Can you work these out from the model? Positions are in its coordinate system, mm. Face numbers are marked on the shaded views. A direction names the side the tool comes from. Coordinates: 2 decimals unless noted, no trailing zeros. Order: outer loops, then holes, each group sorted by start corner. A loop starts at its lowest first (then second) coordinate and runs counter-clockwise, first axis right, second up. Notation, with made-up numbers: (-18.5, -26) -> (5.5, -26) arc R14 ccw to (5.5, -8) -> close; hole circle Ø1 at (-25.5, 56.5). An arc over 180 degrees is marked (long way). Write item = value, one per line.
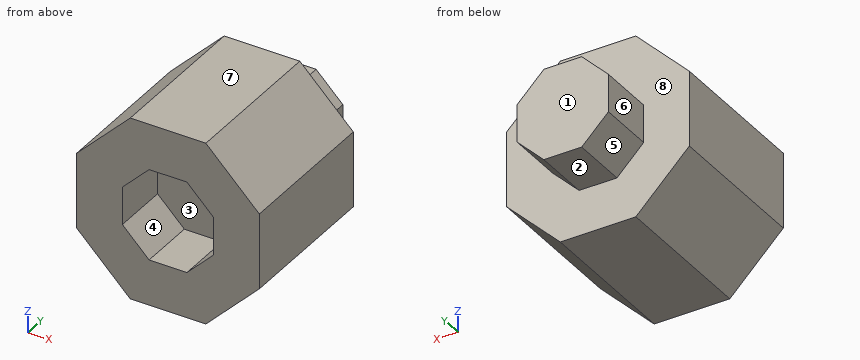
```python
from build123d import *

# Parameters (mm, degrees)
F1_DEPTH = 40
F3_DEPTH = 15
F5_DEPTH = 15


with BuildPart() as f1:
    # F0 (on Front) → F1 (new body)
    with BuildSketch(Plane.XZ):
        Polygon((24, -9.941125497), (24, 9.941125497), (9.941125497, 24), (-9.941125497, 24), (-24, 9.941125497), (-24, -9.941125497), (-9.941125497, -24), (9.941125497, -24), align=None)
    extrude(amount=F1_DEPTH)

    # F2 (on Front) → F3 (join)
    with BuildSketch(Plane.XZ):
        Polygon((4.9705627485, -12), (12, -4.9705627485), (12, 4.9705627485), (4.9705627485, 12), (-4.9705627485, 12), (-12, 4.9705627485), (-12, -4.9705627485), (-4.9705627485, -12), align=None)
    extrude(amount=-F3_DEPTH)

    # F4 (on face) → F5 (cut)
    with BuildSketch(Plane.XZ.offset(40)):
        Polygon((-4.9705627485, -12), (4.9705627485, -12), (12, -4.9705627485), (12, 4.9705627485), (4.9705627485, 12), (-4.9705627485, 12), (-12, 4.9705627485), (-12, -4.9705627485), align=None)
    extrude(amount=-F5_DEPTH, mode=Mode.SUBTRACT)


solid = f1.part
```
Item 1: For the marked faces 4, 5, 6, 7 and 8, which set-ups out of +Z, -Z, +X, -X, +Y, -Y let a thin tool reach every point of the face, with its end or its side?
A:
face_4 = -Y
face_5 = -Z, -X, +Y
face_6 = +Z, -Z, -X, +Y
face_7 = +Z, +X, -X, +Y, -Y
face_8 = +Y
Item 2: I want a section at B-B, the plane x = 1. Please give me the cut outline in (y, z), plus the area to 3 significant figures.
A:
outline = (-40, -24) -> (0, -24) -> (0, -12) -> (15, -12) -> (15, 12) -> (0, 12) -> (0, 24) -> (-40, 24) -> (-40, 12) -> (-25, 12) -> (-25, -12) -> (-40, -12) -> close
area = 1,920 mm2
Item 3: If we mould it in two halves opening along Z, with no side actions, what happens to the marked faces 1, 2 and 3? For each: pulls with the +Z half, pulls with the -Z half, needs draft (parallel to the pull), parting line crosses it, or undercut.
A:
face_1 = needs draft
face_2 = pulls with the -Z half
face_3 = undercut
Item 4: I'm going to push flat-ended pins straight in: P1, Ø5, axis at y = 5.5, z = -1.5, coming from the +X side; P2, Ø11, axis at y = 8, z = 0, coming from the -X side; P3, Ø6, axis at x = -11, y = -33, coming from the +Z side; P4, Ø3, axis at y = -11.5, z = -13.5, coming from the -X side. Where does each tip first touch, or does it pass through?
A:
P1 = 12
P2 = -12
P3 = 24
P4 = -21.94
Item 5: I want a section at C-C, the plane y = 10. Please give me the cut outline in (x, z), plus the area to 3 significant figures.
A:
outline = (-12, -4.97) -> (-4.97, -12) -> (4.97, -12) -> (12, -4.97) -> (12, 4.97) -> (4.97, 12) -> (-4.97, 12) -> (-12, 4.97) -> close
area = 477 mm2
Item 6: If I drill on probe 1 along X at (y, z) = (-29, 1.5); probe 2 along Y at (x, z) = (-8, -5); probe 3 along Y at (x, z) = (-14, -18), over which ranges is the centre line in solid material (lowest first)?
A:
probe_1 = -24 to -12, 12 to 24
probe_2 = -25 to 15
probe_3 = -40 to 0
Item 7: I want a section at A-A, the plane y = -27. Please give me the cut outline in (x, z), plus the area to 3 significant figures.
A:
outline = (-24, -9.94) -> (-9.94, -24) -> (9.94, -24) -> (24, -9.94) -> (24, 9.94) -> (9.94, 24) -> (-9.94, 24) -> (-24, 9.94) -> close; hole (-12, -4.97) -> (-4.97, -12) -> (4.97, -12) -> (12, -4.97) -> (12, 4.97) -> (4.97, 12) -> (-4.97, 12) -> (-12, 4.97) -> close
area = 1,430 mm2
Item 8: I want a section at D-D, the plane z = -2. Please give me the cut outline in (x, y), plus the area to 3 significant figures.
A:
outline = (-24, -40) -> (-12, -40) -> (-12, -25) -> (12, -25) -> (12, -40) -> (24, -40) -> (24, 0) -> (12, 0) -> (12, 15) -> (-12, 15) -> (-12, 0) -> (-24, 0) -> close
area = 1,920 mm2
